Geometry: see drawing. Coordinates: mm, zero at the bounding-box minimum. A direction names the side the tool comes from. Coordinates: 2 decimals unless noted, no trailing zeros. Order: outer loops, then holes, each group sorted by start corner. A loop starts at its lowest first (then second) coordinate and runs counter-clockwise, first axis right, second up.
Item 1: Ray query, line 1 (Z direction, x = 5.5, y = 35.5); line 2 (Y direction, x = 20.5, z = 48). Return the intervals inside material, ascending.
Item 2: Section C-C on z = 50. Return the cut outline in (x, y), then the cut area to 3 significant figures.
Item 3: Reachability of the marked faces 1 and 2 from +Z, -Z, +X, -X, +Y, -Y: full face, straight path, thin tool, end or side. Return the list, or none.
Item 4: Section A-A on x = 21.15. Return the cut outline in (y, z).
Item 5: Contact query for a flat-ended pin moving along its axis: P1, Ø1.5, axis at x = 24, z = 43.5, coming from the +Y side. Output: stop coordinate, or through.
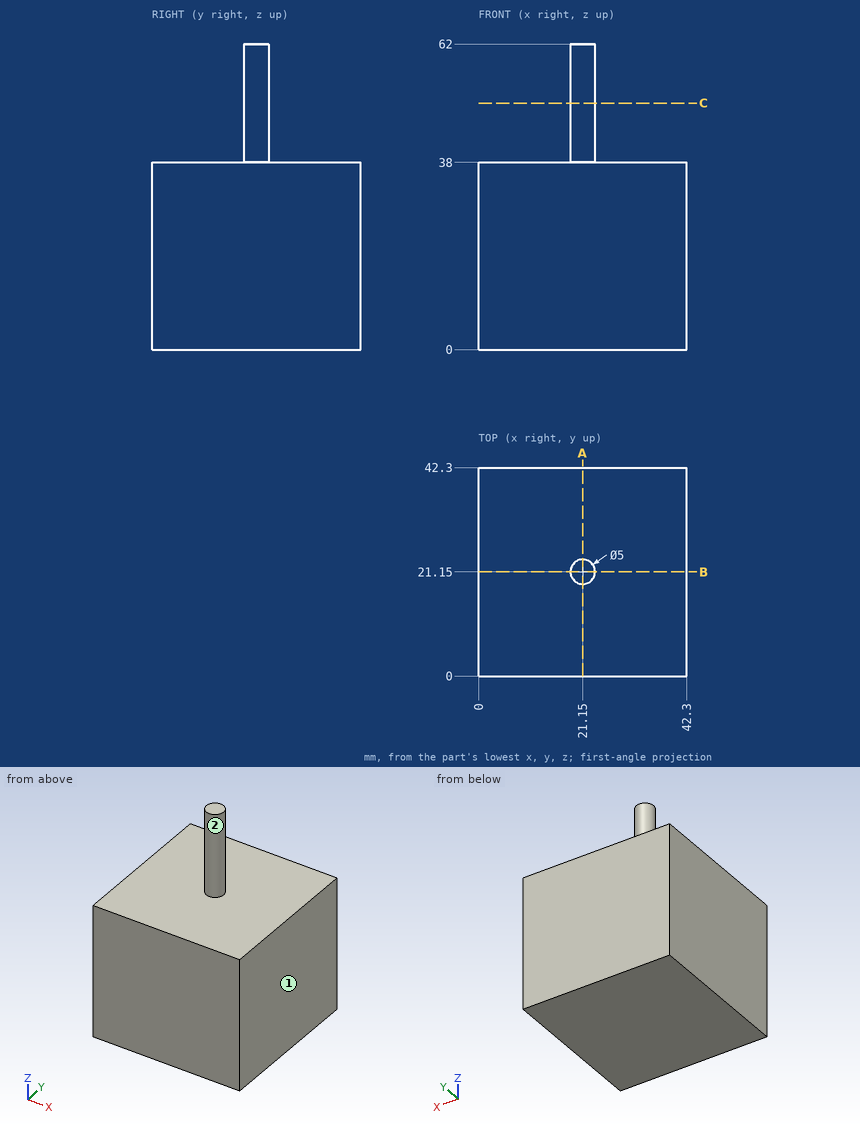
Answer list:
1. line 1: z = 0 to 38
1. line 2: y = 18.74 to 23.56
2. outline: circle Ø5 at (21.15, 21.15)
2. area: 19.6 mm2
3. face 1: +Z, -Z, +X, +Y, -Y
3. face 2: +Z
4. outline: (0, 0) - (42.3, 0) - (42.3, 38) - (23.65, 38) - (23.65, 62) - (18.65, 62) - (18.65, 38) - (0, 38) - close
5. P1: stops at y = 22.51
